Here's how the part is built. I have some questions about the finished solid (model axes, mm). Face numbers are marked on the shaded views. A direction names the side the tool comes from. Coordinates: 2 decimals unless noted, no trailing zeros. Write each loop counter-clockwise with the first axis right and the second up, starting at its lowest first coordinate (ties: lowest second). Pieces come first, ordered by that corner, then holes. Notation, with made-up numbers: (6, 67) -> (38, 67) arc R8 cw to (38, 76) -> close; hole circle Ø7 at (-20.75, -11.5). An arc over 180 degrees is marked (long way). Use a Markdown table: item, result. Add a question column.
Item 1: On a 3-axis mill with a long thin cutter (end or side, diameter ignored), from which of +Z, -Z, +X, -X, +Y, -Y can I reach the whole of each face in a straight line? I mean the marked faces 1 and 2. Say none if no direction works.
Item 2: If I drill on line 1 along X through (y, z) = (1, 36) (3 decimals); line 2 along Y through (x, z) = (2, 62.5); line 3 along Z through (x, y) = (13.5, 41), over which ranges is the centre line in solid material (lowest first)? Write a range as from..to.
Item 3: Will these pins go through, and if not, where does the flat tip stop? pin 1 Ø10 at (x, z) = (-9, 36) entering from -Y; pin 2 Ø8 at (x, z) = (12.5, 53.5) entering from +Y; pin 3 Ø12 at (x, y) = (-0.5, -11.5) entering from +Z.
Item 4: Imagine slicing it at A-A, the plane z = 24.5. Write out the boundary of the cut face in (x, y) (3 decimals).
Item 5: If we mould it in two halves opening along X, with no side actions, what happens to the marked faces 3, 4 and 5? For each: pulls with the +X half, pulls with the -X half, needs draft (parallel to the pull), parting line crosses it, or undercut.
```python
from build123d import *

# Parameters (mm, degrees)
F0_W     = 44.45
F0_H     = 101.6
F1_DEPTH = 101.6
F2_R     = 19.05
F3_T     = -2.54
F4_R     = 2.53999


# Not quite as in the source:
# - a fillet or chamfer is up to 0.001 mm smaller than in the source, because OpenCascade refuses the exact size


with BuildPart() as f1:
    # F0 (on Top) → F1 (new body)
    with BuildSketch(Plane.XY):
        Rectangle(F0_W, F0_H)
    extrude(amount=F1_DEPTH)

    # F2
    f2_edges = [f1.edges().sort_by_distance(p)[0] for p in [
        (-22.225, 50.8, 50.8),
        (-22.225, -50.8, 50.8),
        (22.225, -50.8, 50.8),
        (22.225, 50.8, 50.8),
    ]]
    fillet(f2_edges, radius=F2_R)

    # F3
    f3_openings = [f1.faces().sort_by_distance(p)[0] for p in [
        (0, 0, 101.6),
    ]]
    offset(amount=F3_T, openings=f3_openings)

    # F4 (radius 2.54 in the source; OpenCascade refuses exactly that, so slightly less here)
    f4_edges = [f1.edges().sort_by_distance(p)[0] for p in [
        (22.225, 0, 0),
        (22.225, -31.75, 50.8),
        (22.225, 31.75, 50.8),
        (22.225, 0, 101.6),
        (-22.225, 0, 0),
        (-22.225, 31.75, 50.8),
        (-22.225, -31.75, 50.8),
        (-22.225, 0, 101.6),
    ]]
    fillet(f4_edges, radius=F4_R)


solid = f1.part
```
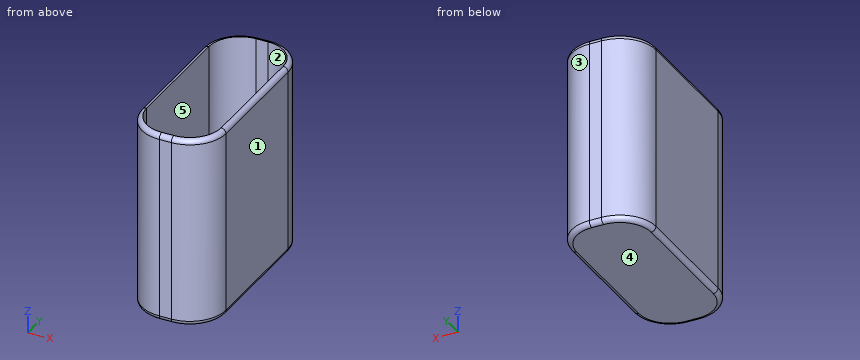
Ans:
| question | item | result |
|---|---|---|
| 1 | face 1 | +Z, -Z, +X, +Y, -Y |
| 1 | face 2 | +Z |
| 2 | line 1 | x = -22.225..-19.685, 19.685..22.225 |
| 2 | line 2 | y = -50.8..-48.26, 48.26..50.8 |
| 2 | line 3 | z = 0..2.54 |
| 3 | pin 1 | stops at y = -50.78 |
| 3 | pin 2 | stops at y = 50.04 |
| 3 | pin 3 | stops at z = 2.54 |
| 4 | outline | (-22.225, -31.75) arc R19.05 ccw to (-3.175, -50.8) -> (3.175, -50.8) arc R19.05 ccw to (22.225, -31.75) -> (22.225, 31.75) arc R19.05 ccw to (3.175, 50.8) -> (-3.175, 50.8) arc R19.05 ccw to (-22.225, 31.75) -> close; hole (-19.685, -31.75) arc R16.51 ccw to (-3.175, -48.26) -> (3.175, -48.26) arc R16.51 ccw to (19.685, -31.75) -> (19.685, 31.75) arc R16.51 ccw to (3.175, 48.26) -> (-3.175, 48.26) arc R16.51 ccw to (-19.685, 31.75) -> close |
| 5 | face 3 | pulls with the +X half |
| 5 | face 4 | needs draft |
| 5 | face 5 | undercut |
